```python
from build123d import *

# Parameters (mm, degrees)
SKETCH_1_R          = 12.5
EXTRUDE_1_DEPTH     = 40
CHAMFER_1_SIZE      = 0.5
CUT_EXTRUDE_1_DEPTH = 4
SKETCH_4_R          = 15
EXTRUDE_2_DEPTH     = 49
CHAMFER_2_SIZE      = 0.5
SKETCH_7_R          = 14.5
EXTRUDE_3_DEPTH     = 2
SKETCH_8_R          = 20
EXTRUDE_4_DEPTH     = 1170
SKETCH_9_R          = 14.5
EXTRUDE_5_DEPTH     = 2
SKETCH_10_R         = 15
EXTRUDE_6_DEPTH     = 47
CHAMFER_3_SIZE      = 0.5


with BuildPart() as part:
    # 草图1 → 凸台-拉伸1 (new body)
    with BuildSketch(Plane.XY):
        Circle(SKETCH_1_R)
    extrude(amount=EXTRUDE_1_DEPTH)

    # 倒角1
    chamfer_1_edges = [part.edges().sort_by_distance(p)[0] for p in [
        (-12.5, 0, 40),
    ]]
    chamfer(chamfer_1_edges, length=CHAMFER_1_SIZE)

    # 草图3 → 切除-拉伸1 (cut)
    with BuildSketch(Plane(origin=(0, 12.5, 0), x_dir=(1, 0, 0), z_dir=(0, 1, 0))):
        with BuildLine():
            Line((4, -11), (4, -33))
            ThreePointArc((4, -33), (0, -37), (-4, -33))
            Line((-4, -33), (-4, -11))
            ThreePointArc((-4, -11), (0, -7), (4, -11))
        make_face()
    extrude(amount=-CUT_EXTRUDE_1_DEPTH, mode=Mode.SUBTRACT)

    # 草图4 → 凸台-拉伸2 (add)
    with BuildSketch(Plane(origin=(0, 0, 0), x_dir=(-1, 0, 0), z_dir=(0, 0, -1))):
        Circle(SKETCH_4_R)
    extrude(amount=EXTRUDE_2_DEPTH)

    # 倒角2
    chamfer_2_edges = [part.edges().sort_by_distance(p)[0] for p in [
        (15, 0, 0),
    ]]
    chamfer(chamfer_2_edges, length=CHAMFER_2_SIZE)

    # 草图7 → 凸台-拉伸3 (add)
    with BuildSketch(Plane(origin=(0, 0, -49), x_dir=(-1, 0, 0), z_dir=(0, 0, -1))):
        Circle(SKETCH_7_R)
    extrude(amount=EXTRUDE_3_DEPTH)

    # 草图8 → 凸台-拉伸4 (add)
    with BuildSketch(Plane(origin=(0, 0, -51), x_dir=(-1, 0, 0), z_dir=(0, 0, -1))):
        Circle(SKETCH_8_R)
    extrude(amount=EXTRUDE_4_DEPTH)

    # 草图9 → 凸台-拉伸5 (add)
    with BuildSketch(Plane(origin=(0, 0, -1221), x_dir=(-1, 0, 0), z_dir=(0, 0, -1))):
        Circle(SKETCH_9_R)
    extrude(amount=EXTRUDE_5_DEPTH)

    # 草图10 → 凸台-拉伸6 (add)
    with BuildSketch(Plane(origin=(0, 0, -1223), x_dir=(-1, 0, 0), z_dir=(0, 0, -1))):
        Circle(SKETCH_10_R)
    extrude(amount=EXTRUDE_6_DEPTH)

    # 倒角3
    chamfer_3_edges = [part.edges().sort_by_distance(p)[0] for p in [
        (15, 0, -1270),
    ]]
    chamfer(chamfer_3_edges, length=CHAMFER_3_SIZE)


solid = part.part
```
Check sheet for the modelled part. Datum: model origin and axes. Units: mm. A direction names the side the tool comes from. Coordinates: 2 decimals unless noted, no trailing zeros. Order: outer loops, then holes, each group sorted by start corner. A loop starts at its lowest first (then second) coordinate and runs counter-clockwise, first axis right, second up. Notation, with made-up numbers: (-16.5, 19.5) -> (30.5, 19.5) arc R11 ccw to (30.5, 37.5) -> close; hole circle Ø3 at (79, 9). An arc over 180 degrees is marked (long way). Write each question's results on one line, items separated by ' | '. Start each with the question number.
1) Depth check by flat-ended pin: pin 1 (2 mm diameter, centred on x = 13, z = -960.5, fed in from +Y); pin 2 (1.5 mm diameter, centred on x = 10, z = -149, fed in from -Y); pin 3 (1 mm diameter, centred on y = 11, z = 20.5, fed in from +X). Enter the tip coordinate at first touch or a pass-through.
2) Set-up check for faces 1 (the face through (0, 0, -1270)), 2 (the face through (11, 7, 0)): record each of +Z, -Z, +X, -X, +Y, -Y from which the full face is reachable in a straight line by a thin tool's end or side.
3) Material ranges on line 1 along Z through (x, y) = (-14.5, 2.5); line 2 along X through (y, z) = (15.5, -994.5); line 3 along Z through (x, y) = (-1.5, 17), recorded low to high.
4) Section check B-B (z = -955). Enter the section's corners in (x, y).
Checked values:
1) pin 1: y = 16 | pin 2: y = -17.73 | pin 3: x = 6.78
2) face 1: -Z, +X, -X, +Y, -Y | face 2: +Z
3) line 1: -1269.79 to -1223, -1221 to -51, -49 to -0.21 | line 2: -12.64 to 12.64 | line 3: -1221 to -51
4) outline: circle Ø40 at (0, 0)
